from build123d import *

# Parameters (mm, degrees)
SKETCH1_W           = 20
SKETCH1_H           = 12
BOSS_EXTRUDE1_DEPTH = 10
SKETCH4_R           = 3
BOSS_EXTRUDE2_DEPTH = 1
FILLET1_R           = 6


with BuildPart() as part:
    # Sketch1 → Boss-Extrude1 (new body)
    with BuildSketch(Plane(origin=(0, 0, 0), x_dir=(1, 0, 0), z_dir=(0, 1, 0))):
        with Locations((0, 6)):
            Rectangle(SKETCH1_W, SKETCH1_H)
    extrude(amount=BOSS_EXTRUDE1_DEPTH)

    # Sketch4 → Boss-Extrude2 (add, symmetric)
    with BuildSketch(Plane(origin=(-6, 0, 0), x_dir=(0, 0, -1), z_dir=(1, 0, 0))):
        with BuildLine():
            Line((2, 10), (2, 20))
            ThreePointArc((2, 20), (7.774808523, 23.807886553), (9, 17))
            Line((9, 17), (9, 10))
            Line((9, 10), (2, 10))
        make_face()
        with Locations((6.142857143, 20)):
            Circle(SKETCH4_R, mode=Mode.SUBTRACT)
    boss_extrude2 = extrude(amount=BOSS_EXTRUDE2_DEPTH, both=True)

    # Mirror1: Boss-Extrude2 across plane
    add(boss_extrude2.mirror(Plane(origin=(0, 0, 0), x_dir=(0, 0, 1), z_dir=(1, 0, 0))))

    # Fillet1
    fillet1_edges = [part.edges().sort_by_distance(p)[0] for p in [
        (-10, 5, -12),
        (10, 5, -12),
        (10, 5, 0),
        (-10, 5, 0),
    ]]
    fillet(fillet1_edges, radius=FILLET1_R - 0.0001)  # a hair under: the kernel refuses the full size


solid = part.part
Geometry: final body of the model. Coordinates: model frame, mm. A direction names the side the tool comes from. Coordinates: 2 decimals unless noted, no trailing zeros. Loops run counter-clockwise (first coordinate to the right, second up) from the corner with the lowest first, then second, coordinate; pieces in that order, holes last. Notation, with made-up numbers: (-31, 27) - (13, 27) arc R17 ccw to (13, 58) - close; hole circle Ø10 at (74, -1). An arc over 180 degrees is marked (long way). Put each result on its own line as item: value. Start each with the question number.
Q1. Cut plane C-C, the plane z = -2.75. Return loops of the section in (x, y).
Q2. Cut plane B-B, the plane z = -4.75. Return loops of the section in (x, y), and give its area (3 significant figures).
Q3. Line query: line 1 (X direction, y = 15.75, z = -2.5); line 2 (Y direction, x = -4.25, z = -5.5); line 3 (Y direction, x = -6.75, z = -8.75). Output: solid intervals per line, ascending.
Q4. Set-up query: faces 5 (the flat face through (6, 14, -9)), 6 (the flat face through (-6, 15, -2)), 7 (the flat face through (-5, 16, -6)), 8 (the flat face through (-7, 16, -6)). Return all of +Z, -Z, +X, -X, +Y, -Y with unobstructed straight access to the full face (end or side cutting, diameter ignored); none if empty.
Q5. Cut plane A-A, the plane y = 11. Return loops of the section in (x, z).
Q6. Cut plane D-D, the plane x = 2.5. Return loops of the section in (y, z), and give its area (3 significant figures).
Q7. Pin query (flat end, axial travel): pin 1 Ø1.6 at (x, y) = (-6.5, 12) entering from -Z; pin 2 Ø1 at (x, z) = (2, -1.5) entering from +Y; pin 3 Ø3.5 at (x, z) = (-4, -3.5) entering from +Y; pin 4 Ø4 at (y, z) = (20, -6) entering from -X. Return the tip coordinate at first contact, or that it passes through.
Q8. Pull-direction query (Z, two-part tool) for faces 1 (the cylindrical face through (8.196, 5.07, -10.289)), 2 (the cylindrical face through (6.01, 17.07, -5.49)), 3 (the flat face through (6, 15, -2)), 4 (the flat face through (5, 16, -6)); classes: released by +Z, released by -Z, zero draft, split by the parting line, or undercut.
Filled sheet:
1. outline: (-9.04, 0) - (9.04, 0) - (9.04, 10) - (7, 10) - (7, 22.38) - (5, 22.38) - (5, 10) - (-5, 10) - (-5, 22.38) - (-7, 22.38) - (-7, 10) - (-9.04, 10) - close
2. outline: (-9.87, 0) - (9.87, 0) - (9.87, 10) - (7, 10) - (7, 17.34) - (5, 17.34) - (5, 10) - (-5, 10) - (-5, 17.34) - (-7, 17.34) - (-7, 10) - (-9.87, 10) - close; (-7, 22.66) - (-5, 22.66) - (-5, 23.9) - (-7, 23.9) - close; (5, 22.66) - (7, 22.66) - (7, 23.9) - (5, 23.9) - close
2. area: 232 mm²
3. line 1: -7 to -5, 5 to 7
3. line 2: 0 to 10
3. line 3: 0 to 18.52, 21.48 to 23.22
4. face 5: -Z, +X, -X
4. face 6: +Z, +X, -X, +Y
4. face 7: +Z, -Z, +Y
4. face 8: +Z, -Z, -X, +Y
5. outline: (-7, -9) - (-5, -9) - (-5, -2) - (-7, -2) - close; (5, -9) - (7, -9) - (7, -2) - (5, -2) - close
6. outline: (0, -12) - (10, -12) - (10, 0) - (0, 0) - close
6. area: 120 mm²
7. pin 1: z = -9
7. pin 2: y = 10
7. pin 3: y = 23.96
7. pin 4: through
8. face 1: released by -Z
8. face 2: undercut
8. face 3: released by +Z
8. face 4: zero draft
